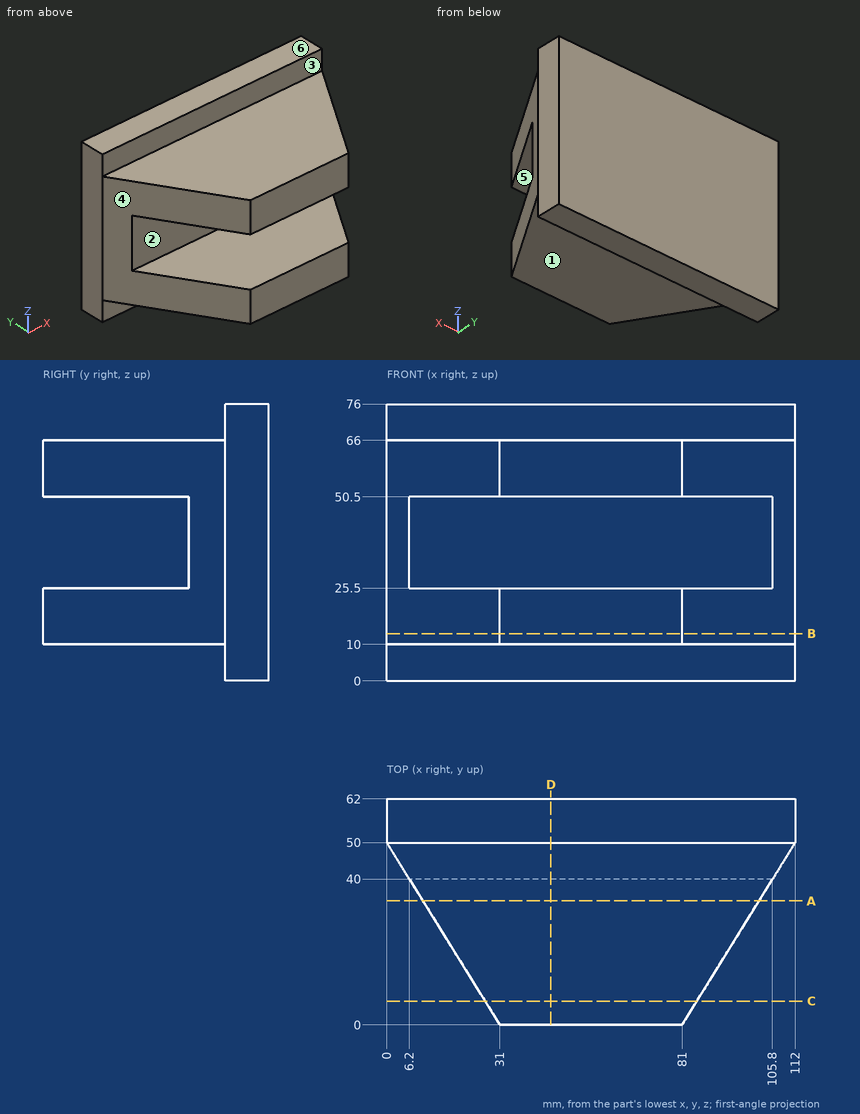
Print and shaded views of the part. All mm, measured from the part's lowest x, y and z. A direction names the side the tool comes from. Round coordinates to 2 decimals unless told otherwise and drop trailing zeros. Order: outer loops, then holes, each group sorted by start corner. A loop starts at its lowest first (then second) coordinate and runs counter-clockwise, first axis right, second up. Notation, with made-up numbers: (77, 36.25) - (107, 36.25) arc R25 ccw to (107, 59.25) - close; hole circle Ø8 at (-26.5, 5). An arc over 180 degrees is marked (long way). Use a Markdown table: item, result.
1) Flat gauge pins, fed straight in: pin 1 Ø25 at (x, y) = (65.5, 14.5) entering from -Z; pin 2 Ø12 at (x, z) = (46.5, 35) entering from -Y; pin 3 Ø8 at (x, z) = (29, 69) entering from -Y; pin 4 Ø4 at (x, z) = (11.5, 21) entering from -Y. Where does each tip first touch, or does it go through?
Recorded:
| item | result |
|---|---|
| pin 1 | stops at z = 10 |
| pin 2 | stops at y = 40 |
| pin 3 | stops at y = 0 |
| pin 4 | stops at y = 28.23 |
2) Wall check: L1, parallel to Z at x = 15.5, y = 36; L2, parallel to Y at x = 102.5, z = 35; L3, parallel to Z at x = 79, y = 46.5. Give the ranges that are in metal, low to high.
Recorded:
| item | result |
|---|---|
| L1 | z = 10 to 25.5, 50.5 to 66 |
| L2 | y = 40 to 62 |
| L3 | z = 10 to 66 |
3) Saw through at C-C on y = 6.5. Write the cut outline in (x, z), and give its area (3 significant figures).
Recorded:
| item | result |
|---|---|
| outline | (26.97, 10) - (85.03, 10) - (85.03, 25.5) - (26.97, 25.5) - close; (26.97, 50.5) - (85.03, 50.5) - (85.03, 66) - (26.97, 66) - close |
| area | 1,800 mm² |
4) Saw through at A-A on y = 34. Write the cut outline in (x, z), and give its area (3 significant figures).
Recorded:
| item | result |
|---|---|
| outline | (9.92, 10) - (102.08, 10) - (102.08, 25.5) - (9.92, 25.5) - close; (9.92, 50.5) - (102.08, 50.5) - (102.08, 66) - (9.92, 66) - close |
| area | 2,860 mm² |
5) Saw through at B-B on z = 13. Write the cut outline in (x, y), and give its area (3 significant figures).
Recorded:
| item | result |
|---|---|
| outline | (0, 50) - (31, 0) - (81, 0) - (112, 50) - (112, 62) - (0, 62) - close |
| area | 5,390 mm² |
6) Saw through at D-D on x = 45. Write the cut outline in (y, z), and give its area (3 significant figures).
Recorded:
| item | result |
|---|---|
| outline | (0, 10) - (50, 10) - (50, 0) - (62, 0) - (62, 76) - (50, 76) - (50, 66) - (0, 66) - (0, 50.5) - (40, 50.5) - (40, 25.5) - (0, 25.5) - close |
| area | 2,710 mm² |
7) Tool access for the marked faces 1, 2 and 3: list every direction of +Z, -Z, +X, -X, +Y, -Y with a clear straight run to the whole face (end or side of a thin tool).
Recorded:
| item | result |
|---|---|
| face 1 | -Z, +X, -X, -Y |
| face 2 | +X, -X, -Y |
| face 3 | +Z, +X, -X, -Y |
8) Pull direction Z, two halves, no side cores. Call the marked faces 4, 5 and 6: pulls with the +Z half, pulls with the -Z half, needs draft (parallel to the pull), parting line crosses it, or undercut.
Recorded:
| item | result |
|---|---|
| face 4 | needs draft |
| face 5 | undercut |
| face 6 | pulls with the +Z half |
